Geometry: final body of the model. Coordinates: model frame, mm. Face numbers are marked on the shaded views. A direction names the side the tool comes from. Round coordinates to 2 decimals unless told otherwise and drop trailing zeros. Loops run counter-clockwise (first coordinate to the right, second up) from the corner with the lowest first, then second, coordinate; pieces in that order, holes last. Notation, with made-up numbers: (43, 78.25) - (68, 78.25) arc R22 ccw to (68, 103.25) - close; hole circle Ø11 at (69, 78). An arc over 180 degrees is marked (long way). Answer in a Markdown table with one row per item. Add a question column.
from build123d import *

# Parameters (mm, degrees)
BOX754_W                     = 6
BOX754_H                     = 6
BOX754_DEPTH                 = 2
BOX756_W                     = 6
BOX756_H                     = 6
BOX756_DEPTH                 = 2
BOX756_PLACEMENT_ANGLE       = 135
BOX753_W                     = 6
BOX753_H                     = 6
BOX753_DEPTH                 = 2
BOX750_W                     = 6
BOX750_H                     = 6
BOX750_DEPTH                 = 2
BOX750_PLACEMENT_ANGLE       = 225
BOX751_W                     = 6
BOX751_H                     = 6
BOX751_DEPTH                 = 2
BOX752_W                     = 6
BOX752_H                     = 6
BOX752_DEPTH                 = 2
BOX752_PLACEMENT_ANGLE       = 45
BOX757_W                     = 6
BOX757_H                     = 6
BOX757_DEPTH                 = 2
BOX749_W                     = 6
BOX749_H                     = 6
BOX749_DEPTH                 = 2
BOX749_PLACEMENT_ANGLE       = 45
CYLINDER1963_R               = 1.5
CYLINDER1963_DEPTH           = 10
CYLINDER1962_R               = 1.5
CYLINDER1962_DEPTH           = 10
CYLINDER1962_PLACEMENT_ANGLE = 135
CYLINDER1954_R               = 1.5
CYLINDER1954_DEPTH           = 10
CYLINDER1952_R               = 1.5
CYLINDER1952_DEPTH           = 10
CYLINDER1952_PLACEMENT_ANGLE = 225
CYLINDER1955_R               = 1.5
CYLINDER1955_DEPTH           = 10
CYLINDER1950_R               = 1.5
CYLINDER1950_DEPTH           = 10
CYLINDER1950_PLACEMENT_ANGLE = 45
CYLINDER1960_R               = 1.5
CYLINDER1960_DEPTH           = 10
CYLINDER1961_R               = 1.5
CYLINDER1961_DEPTH           = 10
CYLINDER1961_PLACEMENT_ANGLE = 45
CYLINDER1956_R               = 2.2
CYLINDER1956_DEPTH           = 10
TORUS003_R                   = 2.2
TUBE101_R                    = 35
TUBE101_R_2                  = 29
TUBE101_DEPTH                = 20


with BuildPart() as krychle754:
    # Box754 → Box754 (new body)
    with BuildSketch(Plane(origin=(-29, -3, 14), x_dir=(0, 1, 0), z_dir=(0, 0, 1))):
        with Locations((3, 3)):
            Rectangle(BOX754_W, BOX754_H)
    extrude(amount=BOX754_DEPTH)


with BuildPart() as krychle756:
    # Box756 → Box756 (new body)
    with BuildSketch(Plane.XY):
        with Locations((3, 3)):
            Rectangle(BOX756_W, BOX756_H)
    extrude(amount=BOX756_DEPTH)


with BuildPart() as krychle756_1:
    # Box756 placement: moved
    add(krychle756.part.moved(Location((-18.384776, -22.627417, 14))).rotate(Axis((-18.384776, -22.627417, 14), (0, 0, 1)), BOX756_PLACEMENT_ANGLE))


with BuildPart() as krychle753:
    # Box753 → Box753 (new body)
    with BuildSketch(Plane(origin=(3, -29, 14), x_dir=(-1, 0, 0), z_dir=(0, 0, 1))):
        with Locations((3, 3)):
            Rectangle(BOX753_W, BOX753_H)
    extrude(amount=BOX753_DEPTH)


with BuildPart() as krychle750:
    # Box750 → Box750 (new body)
    with BuildSketch(Plane.XY):
        with Locations((3, 3)):
            Rectangle(BOX750_W, BOX750_H)
    extrude(amount=BOX750_DEPTH)


with BuildPart() as krychle750_1:
    # Box750 placement: moved
    add(krychle750.part.moved(Location((22.627417, -18.384776, 14))).rotate(Axis((22.627417, -18.384776, 14), (0, 0, 1)), BOX750_PLACEMENT_ANGLE))


with BuildPart() as krychle751:
    # Box751 → Box751 (new body)
    with BuildSketch(Plane(origin=(29, 3, 14), x_dir=(0, -1, 0), z_dir=(0, 0, 1))):
        with Locations((3, 3)):
            Rectangle(BOX751_W, BOX751_H)
    extrude(amount=BOX751_DEPTH)


with BuildPart() as krychle752:
    # Box752 → Box752 (new body)
    with BuildSketch(Plane.XY):
        with Locations((3, 3)):
            Rectangle(BOX752_W, BOX752_H)
    extrude(amount=BOX752_DEPTH)


with BuildPart() as krychle752_1:
    # Box752 placement: moved
    add(krychle752.part.moved(Location((18.384776, 22.627417, 14))).rotate(Axis((18.384776, 22.627417, 14), (0, 0, -1)), BOX752_PLACEMENT_ANGLE))


with BuildPart() as krychle757:
    # Box757 → Box757 (new body)
    with BuildSketch(Plane(origin=(-3, 29, 14), x_dir=(1, 0, 0), z_dir=(0, 0, 1))):
        with Locations((3, 3)):
            Rectangle(BOX757_W, BOX757_H)
    extrude(amount=BOX757_DEPTH)


with BuildPart() as compound927:
    # Box749 → Box749 (new body)
    with BuildSketch(Plane.XY):
        with Locations((3, 3)):
            Rectangle(BOX749_W, BOX749_H)
    extrude(amount=BOX749_DEPTH)


with BuildPart() as compound927_1:
    # Box749 placement: moved
    add(compound927.part.moved(Location((-22.627417, 18.384776, 14))).rotate(Axis((-22.627417, 18.384776, 14), (0, 0, 1)), BOX749_PLACEMENT_ANGLE))

    # Compound927: union Krychle754, Krychle756, Krychle753, Krychle750, Krychle751, Krychle752, Krychle757
    add(krychle754.part)
    add(krychle756_1.part)
    add(krychle753.part)
    add(krychle750_1.part)
    add(krychle751.part)
    add(krychle752_1.part)
    add(krychle757.part)


with BuildPart() as obj1:
    # Cylinder1963 → Cylinder1963 (new body)
    with BuildSketch(Plane(origin=(-32, 0, 10), x_dir=(0, 1, 0), z_dir=(0, 0, 1))):
        Circle(CYLINDER1963_R)
    extrude(amount=CYLINDER1963_DEPTH)


with BuildPart() as obj2:
    # Cylinder1962 → Cylinder1962 (new body)
    with BuildSketch(Plane.XY):
        Circle(CYLINDER1962_R)
    extrude(amount=CYLINDER1962_DEPTH)


with BuildPart() as obj2_1:
    # Cylinder1962 placement: moved
    add(obj2.part.moved(Location((-22.627417, -22.627417, 10))).rotate(Axis((-22.627417, -22.627417, 10), (0, 0, 1)), CYLINDER1962_PLACEMENT_ANGLE))


with BuildPart() as obj3:
    # Cylinder1954 → Cylinder1954 (new body)
    with BuildSketch(Plane(origin=(0, -32, 10), x_dir=(-1, 0, 0), z_dir=(0, 0, 1))):
        Circle(CYLINDER1954_R)
    extrude(amount=CYLINDER1954_DEPTH)


with BuildPart() as obj4:
    # Cylinder1952 → Cylinder1952 (new body)
    with BuildSketch(Plane.XY):
        Circle(CYLINDER1952_R)
    extrude(amount=CYLINDER1952_DEPTH)


with BuildPart() as obj4_1:
    # Cylinder1952 placement: moved
    add(obj4.part.moved(Location((22.627417, -22.627417, 10))).rotate(Axis((22.627417, -22.627417, 10), (0, 0, 1)), CYLINDER1952_PLACEMENT_ANGLE))


with BuildPart() as obj5:
    # Cylinder1955 → Cylinder1955 (new body)
    with BuildSketch(Plane(origin=(32, 0, 10), x_dir=(0, -1, 0), z_dir=(0, 0, 1))):
        Circle(CYLINDER1955_R)
    extrude(amount=CYLINDER1955_DEPTH)


with BuildPart() as obj6:
    # Cylinder1950 → Cylinder1950 (new body)
    with BuildSketch(Plane.XY):
        Circle(CYLINDER1950_R)
    extrude(amount=CYLINDER1950_DEPTH)


with BuildPart() as obj6_1:
    # Cylinder1950 placement: moved
    add(obj6.part.moved(Location((22.627417, 22.627417, 10))).rotate(Axis((22.627417, 22.627417, 10), (0, 0, -1)), CYLINDER1950_PLACEMENT_ANGLE))


with BuildPart() as obj7:
    # Cylinder1960 → Cylinder1960 (new body)
    with BuildSketch(Plane(origin=(0, 32, 10), x_dir=(1, 0, 0), z_dir=(0, 0, 1))):
        Circle(CYLINDER1960_R)
    extrude(amount=CYLINDER1960_DEPTH)


with BuildPart() as compound929:
    # Cylinder1961 → Cylinder1961 (new body)
    with BuildSketch(Plane.XY):
        Circle(CYLINDER1961_R)
    extrude(amount=CYLINDER1961_DEPTH)


with BuildPart() as compound929_1:
    # Cylinder1961 placement: moved
    add(compound929.part.moved(Location((-22.627417, 22.627417, 10))).rotate(Axis((-22.627417, 22.627417, 10), (0, 0, 1)), CYLINDER1961_PLACEMENT_ANGLE))

    # Compound929: union obj1, obj2, obj3, obj4, obj5, obj6, obj7
    add(obj1.part)
    add(obj2_1.part)
    add(obj3.part)
    add(obj4_1.part)
    add(obj5.part)
    add(obj6_1.part)
    add(obj7.part)


with BuildPart() as obj8:
    # Cylinder1956 → Cylinder1956 (new body)
    with BuildSketch(Plane(origin=(28, 0, 20.5), x_dir=(1, 0, 0), z_dir=(0, 0, 1))):
        Circle(CYLINDER1956_R)
    extrude(amount=CYLINDER1956_DEPTH)


with BuildPart() as obj9:
    # Torus003 → Torus003 (revolve)
    with BuildSketch(Plane(origin=(0, 0, 20.5), x_dir=(1, 0, 0), z_dir=(0, -1, 0))):
        with Locations((28, 0)):
            Circle(TORUS003_R)
    revolve(axis=Axis((0, 0, 20.5), (0, 0, 1)))


with BuildPart() as obj10:
    # Tube101 → Tube101 (new body)
    with BuildSketch(Plane.XY.offset(10)):
        Circle(TUBE101_R)
        Circle(TUBE101_R_2, mode=Mode.SUBTRACT)
    extrude(amount=TUBE101_DEPTH)

    # Cut580: cut obj9
    add(obj9.part, mode=Mode.SUBTRACT)

    # Cut582: cut obj8
    add(obj8.part, mode=Mode.SUBTRACT)

    # Cut579: cut Compound929
    add(compound929_1.part, mode=Mode.SUBTRACT)

    # Cut575: cut Compound927
    add(compound927_1.part, mode=Mode.SUBTRACT)


solid = obj10.part
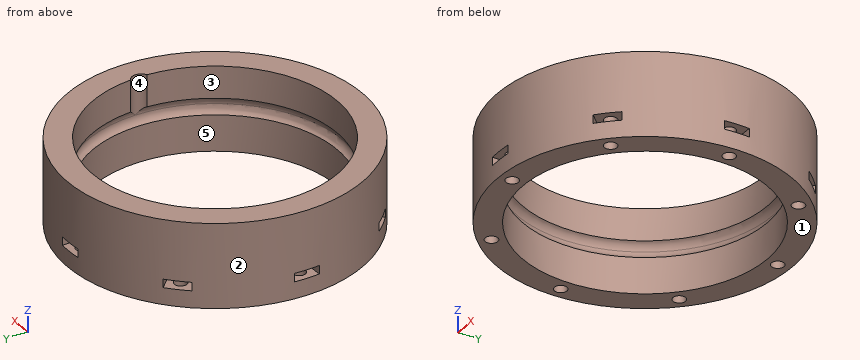
1) Reachability of the marked faces 4 and 5 from +Z, -Z, +X, -X, +Y, -Y: full face, straight path, thin tool, end or side. Return the list, or none.
2) Section C-C, the plane z = 21.5. Return the cut outline in (x, y).
3) Section B-B, the plane y = -32. Return the cut outline in (x, z).
4) Section A-A, the plane x = 19.5. Give the number of separate pieces and of enclosed holes in the cut face, and give its area (3 significant figures).
5) Contact query for flat-ended pins moving along their axis: pin 1 Ø8 at (x, z) = (-21.5, 22.5) entering from +Y; pin 2 Ø1 at (x, z) = (23.5, 26.5) entering from +Y; pin 3 Ø3.5 at (x, y) = (31.5, 0) entering from -Z; pin 4 Ø1 at (y, z) = (-15, 28) entering from +X. Output: stop coordinate, or through.
6) Material intervals for line 1 along X through (y, z) = (0, 16.9); line 2 along Z through (x, y) = (-24, 24); line 3 along X through (y, z) = (0, 27.25), sorted ascending. Write a range as from..to.
7) Pull-direction query (Y, two-part tool) for the marked faces 1, 2 and 3; classes: pulls with the +Y half, pulls with the -Y half, needs draft (parallel to the pull), parting line crosses it, or undercut.
Evaluation:
| question | item | result |
|---|---|---|
| 1 | face 4 | +Z |
| 1 | face 5 | +Z, -Z |
| 2 | outline | circle Ø70 at (0, 0); hole (29.94, -1.03) arc R2.2 ccw to (29.94, 1.03) arc R29.96 ccw (long way) to start |
| 3 | outline | (-14.18, 10) - (-1.5, 10) - (-1.5, 14) - (-3, 14) - (-3, 16) - (-1.5, 16) - (-1.5, 20) - (1.5, 20) - (1.5, 16) - (3, 16) - (3, 14) - (1.5, 14) - (1.5, 10) - (14.18, 10) - (14.18, 30) - (-14.18, 30) - close |
| 4 | separate pieces | 2 |
| 4 | enclosed holes | 2 |
| 4 | area | 286 mm² |
| 5 | pin 1 | stops at y = 30.31 |
| 5 | pin 2 | stops at y = 26.38 |
| 5 | pin 3 | stops at z = 10 |
| 5 | pin 4 | stops at x = 31.86 |
| 6 | line 1 | x = -35..-33.5, -30.5..-29, 29..30.5, 33.5..35 |
| 6 | line 2 | z = 10..14, 16..30 |
| 6 | line 3 | x = -35..-29, 30.2..35 |
| 7 | face 1 | needs draft |
| 7 | face 2 | parting line crosses it |
| 7 | face 3 | undercut |
